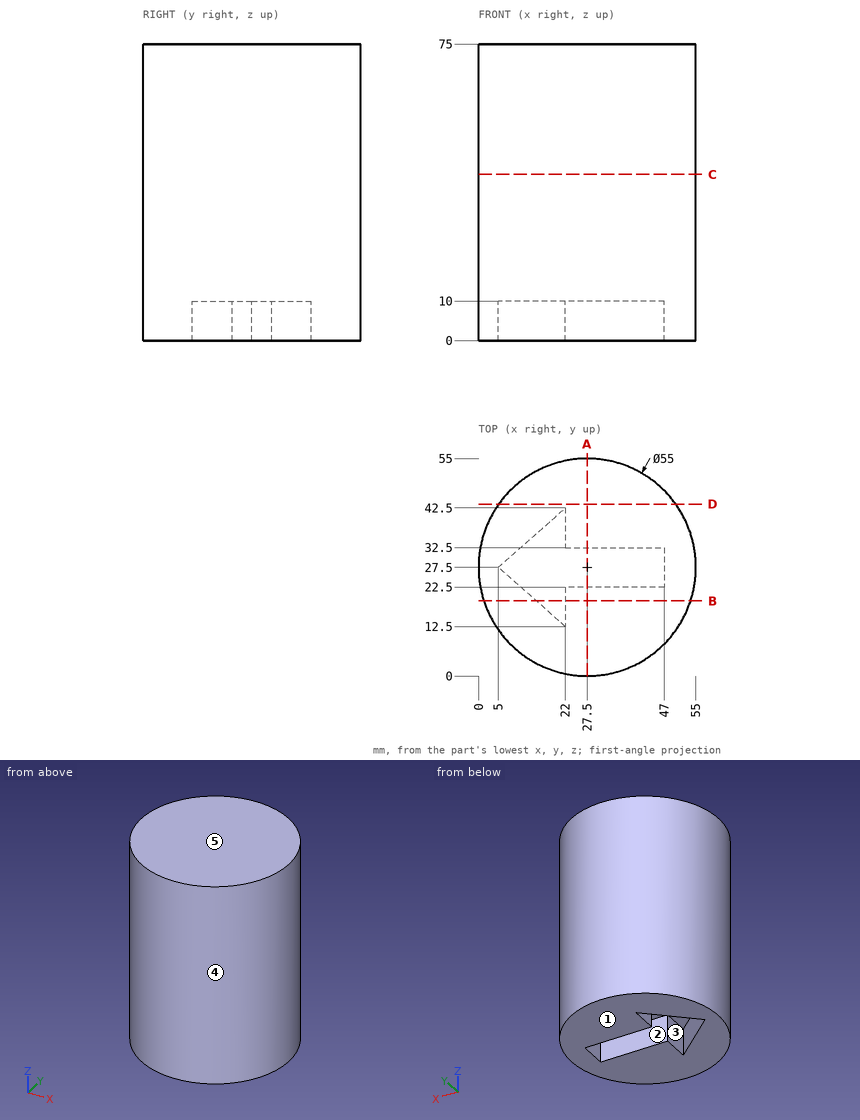
Answer from the drawing. Dimensions are ordinates in mm from the lowest x, y and z of the part. A direction names the side the tool comes from. Coordinates: 2 decimals unless noted, no trailing zeros. Write each loop counter-clockwise with the first axis right and the second up, starting at its lowest first coordinate (ties: lowest second). Pieces come first, ordered by that corner, then holes. Notation, with made-up numbers: (7.5, -33.5) - (35.5, -33.5) arc R23 cw to (35.5, -8.5) - close; hole circle Ø3 at (47.5, -19.5). An arc over 180 degrees is marked (long way). Return JSON: item names as keys, results as strings. Group by question number.
Q1. The part is cut by section B-B on y = 19. Write down the section's boundary in (x, z), and give its area (3 significant figures).
Q2. The part is cut by section C-C on z = 42. Write down the section's boundary in (x, y), and give its area (3 significant figures).
Q3. For a pull along Y with two mould halves and no side action, classify the marked faces 3, 4 and 5 as +Y half, -Y half, draft (parallel to the pull), parting line (faces both ways), or undercut.
Q4. The part is cut by section A-A on x = 27.5. Write down the section's boundary in (y, z), and give its area (4 significant figures).
Q5. Flat-ended cylindrical pins translate along their axes: pin 1 Ø3 at (x, z) = (36.5, 6.5) entering from +Y; pin 2 Ø12 at (x, z) = (41.5, 20.5) entering from +Y; pin 3 Ø2 at (x, z) = (12, 27) entering from +Y. Find the tip coordinate at first contact, or state that the pin passes through.
Q6. Which of the six approach directions +Z, -Z, +X, -X, +Y, -Y give full straight-line access (tool end or side, diameter ignored) to the marked faces 1 and 2?
Q7. Find the intervals of material crossed by line 1 along Z through (x, y) = (31.5, 25); line 2 along Y through (x, z) = (26.5, 41); line 3 along X through (y, z) = (25, 50), in increasing order. Write a range as [from, to].
Q8. The part is cut by section D-D on y = 43.5. Write down the section's boundary in (x, z), and give its area (3 significant figures).
Evaluation:
{
 "1": {"outline": "(1.35, 0) - (14.63, 0) - (14.63, 10) - (22, 10) - (22, 0) - (53.65, 0) - (53.65, 75) - (1.35, 75) - close", "area": "3,850 mm2"},
 "2": {"outline": "circle Ø55 at (27.5, 27.5)", "area": "2,380 mm2"},
 "3": {"face 3": "undercut", "face 4": "parting line", "face 5": "draft"},
 "4": {"outline": "(0, 0) - (22.5, 0) - (22.5, 10) - (32.5, 10) - (32.5, 0) - (55, 0) - (55, 75) - (0, 75) - close", "area": "4,025 mm2"},
 "5": {"pin 1": "stops at y = 53.96", "pin 2": "stops at y = 53.81", "pin 3": "stops at y = 50.87"},
 "6": {"face 1": "-Z, +X, -X, +Y, -Y", "face 2": "-Z"},
 "7": {"line 1": "z = [10, 75]", "line 2": "y = [0.02, 54.98]", "line 3": "x = [0.11, 54.89]"},
 "8": {"outline": "(5.13, 0) - (49.87, 0) - (49.87, 75) - (5.13, 75) - close", "area": "3,350 mm2"}
}
